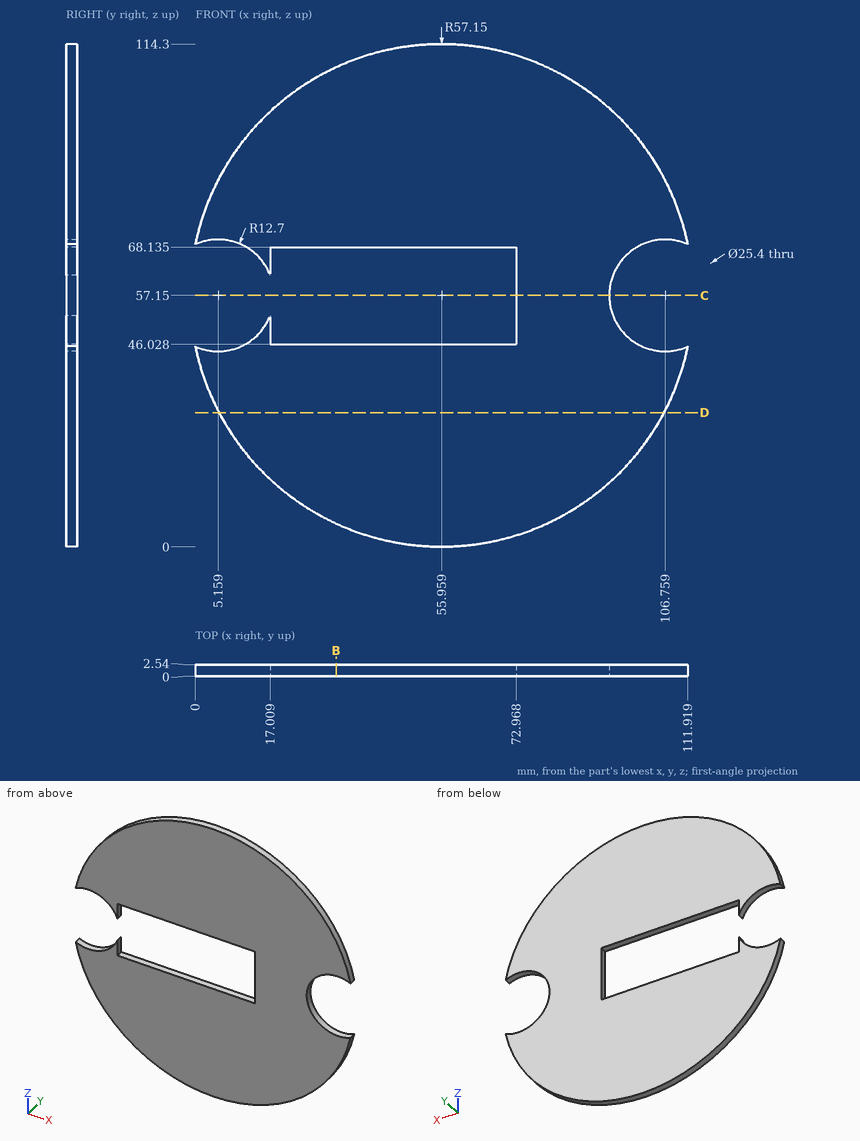
The figure shows three views and two pictorial views of one solid part (mm, origin at its lowest corner). Answer the questions. Coordinates: 2 decimals unless noted, no trailing zeros. Loops run counter-clockwise (first coordinate to the right, second up) from the corner with the lowest first, then second, coordinate; pieces in that order, holes last.
(1) The part is cut by section D-D (z = 30.5). Determine the outline of the cut face in (x, y) (1 decimal).
Solution:
outline: (5.4, 0) - (106.5, 0) - (106.5, 2.5) - (5.4, 2.5) - close
(2) The part is cut by section C-C (z = 57.15). Determine the outline of the cut face in (x, y).
Solution:
outline: (72.97, 0) - (94.06, 0) - (94.06, 2.54) - (72.97, 2.54) - close
(3) The part is cut by section B-B (x = 32). Determine the outline of the cut face in (y, z) (1 decimal).
Solution:
outline: (0, 5.3) - (2.5, 5.3) - (2.5, 46) - (0, 46) - close; (0, 68.1) - (2.5, 68.1) - (2.5, 109) - (0, 109) - close
(4) Flat-ended cylindrical pins translate along their axes: pin 1 Ø0.8 at (y, z) = (1, 49.5) entering from +X; pin 2 Ø1 at (y, z) = (1.5, 12.5) entering from +X; pin 3 Ø0.8 at (x, y) = (35.5, 1) entering from -Z. Find the tip coordinate at first contact, or state that the pin passes through.
Solution:
pin 1: stops at x = 96.94
pin 2: stops at x = 92.25
pin 3: stops at z = 3.64
(5) Consider line 1 along Z through (x, y) = (33.5, 1.35) (1 decimal); line 2 along X through (y, z) = (1.85, 57.15); line 3 along Z through (x, y) = (68, 1.7) (1 decimal). Determine where each line is inside the solid, lowest interval first.
Solution:
line 1: z = 4.6 to 46, 68.1 to 109.7
line 2: x = 72.97 to 94.06
line 3: z = 1.3 to 46, 68.1 to 113
